Here's how the part is built. I have some questions about the finished solid (model axes, mm). A direction names the side the tool comes from. Coordinates: 2 decimals unless noted, no trailing zeros. Write each loop counter-clockwise with the first axis right and the second up, starting at its lowest first coordinate (ties: lowest second). Pieces come first, ordered by that corner, then holes. Notation, with made-up numbers: (-39, 44.25) -> (-21, 44.25) arc R14 ccw to (-21, 68.25) -> close; hole circle Ø3 at (-14.5, 85.25). An arc over 180 degrees is marked (long way). Put each result on its own line as item: value.
Autodesk Inventor part; units mm, degrees
ref_plane "YZ Plane" through (0, 0, 0) normal (1, 0, 0) x (0, 1, 0)
ref_plane "XZ Plane" through (0, 0, 0) normal (0, 1, 0) x (-1, 0, 0)
ref_plane "XY Plane" through (0, 0, 0) normal (0, 0, 1) x (1, 0, 0)
sketch "스케치1" plane through (0, 0, 0) normal (0, 0, 1) x (1, 0, 0)
  line L0 (3.335, 4.5) -> (0, 4.5)
  spline S0 degree 2 poles (3.335, 4.5) (6.7448, 9.4043) (5.1, 12.5) knots 0 0 0 1 1 1
  line L1 (4.5, 3.335) -> (4.5, 0)
  line L2 (-15, 15) -> (-15, -15)
  line L3 (-15, -15) -> (15, -15)
  line L4 (15, -15) -> (-15, 15) construction
  line L5 (-15, -15) -> (15, 15) construction
  line L6 (15, -3.15) -> (12.5, -3.15)
  line L7 (4.5, -3.335) -> (4.5, 0)
  line L8 (12.5, -3.15) -> (12.5, -5.1)
  spline S1 degree 2 poles (4.5, -3.335) (9.4043, -6.7448) (12.5, -5.1) knots 0 0 0 1 1 1
  line L9 (15, -15) -> (15, 15)
  circle A0 centre (10, -10) radius 3
  line L10 (15, 3.15) -> (12.5, 3.15)
  circle A1 centre (10, 10) radius 3
  spline S2 degree 2 poles (4.5, 3.335) (9.4043, 6.7448) (12.5, 5.1) knots 0 0 0 1 1 1
  line L11 (3.15, 12.5) -> (5.1, 12.5)
  line L12 (15, 15) -> (-15, 15)
  line L13 (0, 0) -> (0, 15) construction
  line L14 (3.15, 15) -> (3.15, 12.5)
  line L15 (-3.15, 15) -> (-3.15, 12.5)
  line L16 (-3.15, 12.5) -> (-5.1, 12.5)
  line L17 (-3.335, 4.5) -> (0, 4.5)
  spline S3 degree 2 poles (-3.335, 4.5) (-6.7448, 9.4043) (-5.1, 12.5) knots 0 0 0 1 1 1
  line L18 (-4.5, 3.335) -> (-4.5, 0)
  spline S4 degree 2 poles (-4.5, 3.335) (-9.4043, 6.7448) (-12.5, 5.1) knots 0 0 0 1 1 1
  line L19 (-12.5, 3.15) -> (-12.5, 5.1)
  line L20 (-15, 3.15) -> (-12.5, 3.15)
  circle A2 centre (-10, 10) radius 3
  circle A3 centre (0, 0) radius 2.5
  line L21 (-4.5, -3.335) -> (-4.5, 0)
  line L22 (-15, -3.15) -> (-12.5, -3.15)
  line L23 (-12.5, -3.15) -> (-12.5, -5.1)
  spline S5 degree 2 poles (-4.5, -3.335) (-9.4043, -6.7448) (-12.5, -5.1) knots 0 0 0 1 1 1
  line L24 (-3.335, -4.5) -> (0, -4.5)
  circle A4 centre (-10, -10) radius 3
  line L25 (3.335, -4.5) -> (0, -4.5)
  spline S6 degree 2 poles (-3.335, -4.5) (-6.7448, -9.4043) (-5.1, -12.5) knots 0 0 0 1 1 1
  line L26 (-3.15, -12.5) -> (-5.1, -12.5)
  line L27 (-3.15, -15) -> (-3.15, -12.5)
  spline S7 degree 2 poles (3.335, -4.5) (6.7448, -9.4043) (5.1, -12.5) knots 0 0 0 1 1 1
  line L28 (3.15, -12.5) -> (5.1, -12.5)
  line L29 (3.15, -15) -> (3.15, -12.5)
  line L30 (12.5, 3.15) -> (12.5, 5.1)
  point P0 (5.5866, 9.5531)
  point P1 (9.5531, -5.5866)
  point P2 (9.5531, 5.5866)
  point P3 (-5.5866, 9.5531)
  point P4 (-9.5531, 5.5866)
  point P5 (-9.5531, -5.5866)
  point P6 (-5.5866, -9.5531)
  point P7 (5.5866, -9.5531)
  dimension "d2" = 30
  dimension "d3" = 30
  dimension "d4" = 6
  dimension "d5" = 5
  dimension "d6" = 6.3
  dimension "d7" = 10.2
  dimension "d8" = 6.67
  dimension "d9" = 8
  dimension "d10" = 2.5
  dimension "d11" = 360
  dimension "d12" = 20
extrude "돌출1" add sketch "스케치1" along normal mid plane 158 contours S0 L11 L14 L12 L9 L10 L30 S2 L1 L7 S1 L8 L6 L3 L29 L28 S7 L25 L24 S6 L26 L27 L2 L22 L23 S5 L21 L18 S4 L19 L20 L15 L16 S3 L17 L0
equation "\"TransitionRadius\" = BendRadius"
properties part number "3030 Aluminium Profile 158mm"
Item 1: Imagine slicing it at C-C on z = 8. State how many separate pieces and enclosed holes the cut face has, then the cut area to 3 significant figures.
Output:
separate pieces: 1
enclosed holes: 5
area: 385 mm²
Item 2: If we mould it in two halves opening along Y, with no side actions, what happens to faces 5 (the flat face through (15, -9, -1)), 6 (the flat face through (-4.5, 0, -1)), 7 (the flat face through (-9, -15, -1)), 8 (the cylindrical face through (-12.4, -8.2, -1.1))? For each: released by +Y, released by -Y, zero draft, split by the parting line, or undercut.
Output:
face 5: zero draft
face 6: undercut
face 7: released by -Y
face 8: undercut
Item 3: Which directions (+Z, -Z, +X, -X, +Y, -Y) give clear straight access to the entire face, cutting with the end or side of a thin tool? Please do faces 1 (the flat face through (3.15, -14, -1)), 2 (the flat face through (-3.15, 14, -1)), 3 (the flat face through (9, -15, -1)), 4 (the flat face through (14, -3.15, -1)).
Output:
face 1: +Z, -Z, -Y
face 2: +Z, -Z, +Y
face 3: +Z, -Z, +X, -X, -Y
face 4: +Z, -Z, +X
Item 4: Please list where these lines run through material, in increasing order: line 1 along Y through (x, z) = (10, -34); line 2 along Y through (x, z) = (11, 55.5); line 3 along X through (y, z) = (5, 12). Write a range as from..to.
Output:
line 1: y = -15..-13, -7..-5.63, 5.63..7, 13..15
line 2: y = -15..-12.83, -7.17..-5.59, 5.59..7.17, 12.83..15
line 3: x = -15..-12.5, -7.45..-3.67, 3.67..7.45, 12.5..15
Item 5: For P1, Ø5, axis at y = -3, z = -3, coming from the -X side; P2, Ø2, axis at x = 0, z = 10.5, coming from the -Y side, each with a flat end and sliding along its axis, tell me the tip position at first contact or that it passes through.
Output:
P1: stops at x = -15
P2: stops at y = -4.5
Item 6: Imagine slicing it at A-A on x = 0. Write out the boundary of the cut face in (y, z), then the cut area to 3 significant figures.
Output:
outline: (-4.5, -79) -> (-2.5, -79) -> (-2.5, 79) -> (-4.5, 79) -> close; (2.5, -79) -> (4.5, -79) -> (4.5, 79) -> (2.5, 79) -> close
area: 632 mm²
